Part model, mm, in its own coordinate system. A direction names the side the tool comes from. Give positions to 0.01 mm unless a question says otherwise; leave off trailing zeros. Write each loop counter-clockwise with the first axis right and the second up, starting at its lowest first coordinate (ties: lowest second). Pieces come first, ordered by that corner, then holes. Notation, with made-up numbers: M 89.25,-3.75 L 109.25,-3.75 A21 cw 109.25,10.25 Z; hole C -4,89 d3. An arc over 180 degrees is marked long. Answer as CSV lines item,"result". Start each with the question number.
Item 1: Wall check: L1, parallel to Y at x = 38, z = 31; L2, parallel to Z at x = 209, y = 32; L3, parallel to Y at x = 27, z = 34.5. Give the ranges that are in metal, low to high. Write a range as from..to.
Item 2: Two-plate mould, pull along Z, no slides. Class faces 4 (the flat face through (220, 25, 20)), 5 (the flat face through (108, 32, 34)), 6 (the flat face through (108, 35, 31)), 7 (the flat face through (108, 10, 40)): +Z half, -Z half, draft (parallel to the pull), parting line (faces both ways), or undercut.
Item 3: Pin check, flat tip, straight feed: pin 1 (3 mm diameter, centred on y = 12.5, z = 12, fed in from -X). Stop position of the tip, or through.
Item 4: 3-axis set-ups, long thin cutter, end or side, ignore diameter. For faces 1 (the flat face through (108, 27, 0)), 2 (the flat face through (108, 30, 37)), 3 (the flat face through (108, 25, 28)): which of +Z, -Z, +X, -X, +Y, -Y reach the whole face in a straight line?
Item 5: Band-saw the part on A-A, the plane y = 17. List the corners of the cut face in (x, z).
Item 6: Band-saw the part on B-B, the plane x = 27. List the corners of the cut face in (y, z).
Item 7: Band-saw the part on C-C, the plane y = 27. List the corners of the cut face in (x, z), then the cut area to 3 significant figures.
Item 8: Band-saw the part on D-D, the plane y = 5. List the corners of the cut face in (x, z), then the cut area to 3 significant figures.
from build123d import *

# Parameters (mm, degrees)
F1_DEPTH = 220
F2_R     = 10


with BuildPart() as f1:
    # F0 (on Right) → F1 (new body)
    with BuildSketch(Plane.YZ):
        with BuildLine():
            Line((50, 5), (50, 40))
            Line((50, 40), (30, 40))
            Line((30, 40), (30, 34))
            Line((30, 34), (35, 34))
            Line((35, 34), (35, 28))
            Line((35, 28), (15, 28))
            Line((15, 28), (15, 34))
            Line((15, 34), (20, 34))
            Line((20, 34), (20, 40))
            Line((20, 40), (0, 40))
            Line((0, 40), (0, 0))
            Line((0, 0), (45, 0))
            ThreePointArc((45, 0), (48.535534, 1.464466), (50, 5))
        make_face()
    extrude(amount=F1_DEPTH)

    # F2
    f2_edges = [f1.edges().sort_by_distance(p)[0] for p in [
        (110, 0, 0),
    ]]
    fillet(f2_edges, radius=F2_R)


solid = f1.part
Output:
1,L1,"0..15, 35..50"
1,L2,"0..28, 34..40"
1,L3,"0..20, 30..50"
2,face 4,"draft"
2,face 5,"undercut"
2,face 6,"undercut"
2,face 7,"+Z half"
3,pin 1,"x = 0"
4,face 1,"-Z, +X, -X, +Y, -Y"
4,face 2,"+Z, +X, -X"
4,face 3,"+X, -X"
5,outline,"M 0,0 L 220,0 L 220,28 L 0,28 Z; M 0,34 L 220,34 L 220,40 L 0,40 Z"
6,outline,"M 0,10 A10 ccw 10,0 L 45,0 A5 ccw 50,5 L 50,40 L 30,40 L 30,34 L 35,34 L 35,28 L 15,28 L 15,34 L 20,34 L 20,40 L 0,40 Z"
7,outline,"M 0,0 L 220,0 L 220,28 L 0,28 Z"
7,area,"6,160 mm²"
8,outline,"M 0,1.34 L 220,1.34 L 220,40 L 0,40 Z"
8,area,"8,510 mm²"
